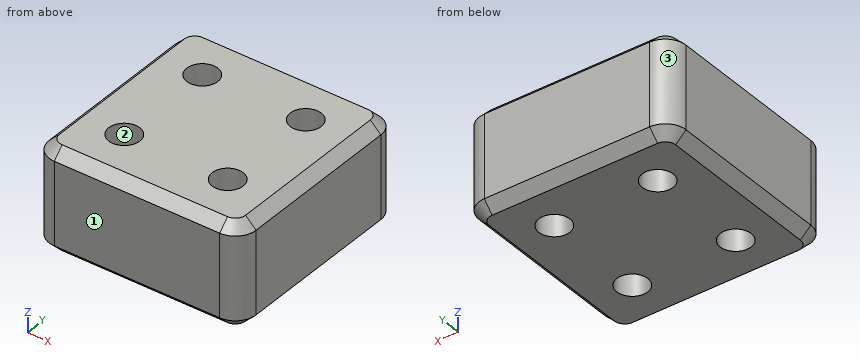
Autodesk Inventor part; units mm, degrees
ref_plane "YZ Plane" through (0, 0, 0) normal (1, 0, 0) x (0, 1, 0)
ref_plane "XZ Plane" through (0, 0, 0) normal (0, 1, 0) x (-1, 0, 0)
ref_plane "XY Plane" through (0, 0, 0) normal (0, 0, 1) x (1, 0, 0)
sketch "스케치1" plane through (0, 0, 0) normal (0, 0, 1) x (1, 0, 0)
  line L0 (-10, -10) -> (10, -10)
  line L1 (10, -10) -> (10, 10)
  line L2 (10, 10) -> (-10, 10)
  line L3 (-10, 10) -> (-10, -10)
  line L4 (-10, -10) -> (10, 10) construction
  line L5 (10, -10) -> (-10, 10) construction
  circle A0 centre (-5, 5) radius 1.5
  circle A1 centre (5, 5) radius 1.5
  circle A2 centre (5, -5) radius 1.5
  circle A3 centre (-5, -5) radius 1.5
  point P0 (0, 0)
  dimension "d0" = 20
  dimension "d1" = 5
  dimension "d2" = 3
extrude "돌출1" add sketch "스케치1" along normal blind 10
fillet "모깎기1" radius 2 4 edges at (-10, 10, 5) (-10, -10, 5) (10, -10, 5) (10, 10, 5)
chamfer "모따기1" distance 1 angle 45 16 edges at (0, 10, 10) (-9.4142, 9.4142, 10) (-10, 0, 10) (-9.4142, -9.4142, 10) (0, -10, 10) (9.4142, -9.4142, 10) (10, 0, 10) (9.4142, 9.4142, 10) (0, 10, 0) (-9.4142, 9.4142, 0) (-10, 0, 0) (-9.4142, -9.4142, 0) (0, -10, 0) (9.4142, -9.4142, 0) (10, 0, 0) (9.4142, 9.4142, 0)
properties part number "RobotBaseConnector_3D 인쇄"
Check sheet for the modelled part. Datum: model origin and axes. Units: mm. Face numbers are marked on the shaded views. Round coordinates to 2 decimals unless told otherwise and drop trailing zeros. Loops run counter-clockwise (first coordinate to the right, second up) from the corner with the lowest first, then second, coordinate; pieces in that order, holes last. Notation, with made-up numbers: (65.5, -24) - (78.5, -24) arc R14 cw to (78.5, 0) - close; hole circle Ø7 at (60, -5). An arc over 180 degrees is marked (long way). Answer as a JSON object with one key per item and string values. Group by question number.
Q1. Mould release check, pull along X, two halves, no side actions. Record for the marked faces 1, 2 and 3: released by +X, released by -X, zero draft, split by the parting line, or undercut.
Q2. Gauge pin test, flat end, axial feed: P1, Ø2.5, axis at x = -5, y = 5, coming from the +Z side. Record the tip position at first contact, or that the pin passes through.
Q3. Sectioned sample at C-C, the plane z = 4.25. Enter the section's corners in (x, y), plus the area to 3 significant figures.
Q4. Sectioned sample at A-A, the plane y = 5. Enter the section's corners in (x, z).
Q5. Scan lines: line 1 along Y through (x, z) = (5, 7.75); line 2 along X through (y, z) = (4, 3); line 3 along Y through (x, z) = (3.75, 6.25). Record each from-to range of solid material in increasing order. Write a range as [from, to].
Solution:
{
 "1": {"face 1": "zero draft", "face 2": "undercut", "face 3": "released by -X"},
 "2": {"P1": "passes through"},
 "3": {"outline": "(-10, -8) arc R2 ccw to (-8, -10) - (8, -10) arc R2 ccw to (10, -8) - (10, 8) arc R2 ccw to (8, 10) - (-8, 10) arc R2 ccw to (-10, 8) - close; hole circle Ø3 at (-5, -5); hole circle Ø3 at (-5, 5); hole circle Ø3 at (5, -5); hole circle Ø3 at (5, 5)", "area": "368 mm²"},
 "4": {"outline": "(-10, 1) - (-9, 0) - (-6.5, 0) - (-6.5, 10) - (-9, 10) - (-10, 9) - close; (-3.5, 0) - (3.5, 0) - (3.5, 10) - (-3.5, 10) - close; (6.5, 0) - (9, 0) - (10, 1) - (10, 9) - (9, 10) - (6.5, 10) - close"},
 "5": {"line 1": "y = [-10, -6.5], [-3.5, 3.5], [6.5, 10]", "line 2": "x = [-10, -6.12], [-3.88, 3.88], [6.12, 10]", "line 3": "y = [-10, -5.83], [-4.17, 4.17], [5.83, 10]"}
}
